```python
from build123d import *

# Parameters (mm, degrees)
SKETCH_1_W          = 20
SKETCH_1_H          = 20
EXTRUDE_1_DEPTH     = 5
SKETCH_2_R          = 1.525
CUT_EXTRUDE_1_DEPTH = 10
CUT_EXTRUDE_2_DEPTH = 6
FILLET_2_R          = 2


with BuildPart() as part:
    # 草图1 → 凸台-拉伸1 (new body)
    with BuildSketch(Plane(origin=(0, 0, 0), x_dir=(1, 0, 0), z_dir=(0, 1, 0))):
        Rectangle(SKETCH_1_W, SKETCH_1_H)
    extrude(amount=EXTRUDE_1_DEPTH)

    # 草图2 → 切除-拉伸1 (cut)
    with BuildSketch(Plane(origin=(0, 5, 0), x_dir=(1, 0, 0), z_dir=(0, 1, 0))):
        with Locations((-7.5, -7)):
            Circle(SKETCH_2_R)
        with Locations((7.5, -7)):
            Circle(SKETCH_2_R)
    extrude(amount=-CUT_EXTRUDE_1_DEPTH, mode=Mode.SUBTRACT)

    # 草图3 → 切除-拉伸2 (cut, through all)
    with BuildSketch(Plane(origin=(0, 5, 0), x_dir=(1, 0, 0), z_dir=(0, 1, 0))):
        Polygon((-10, 10), (-10, 0.585811222), (10, 7.865215908), (10, 10), align=None)
    extrude(amount=-CUT_EXTRUDE_2_DEPTH, mode=Mode.SUBTRACT)

    # 圆角2
    fillet_2_edges = [part.edges().sort_by_distance(p)[0] for p in [
        (-10, 2.5, -0.585811222),
        (10, 2.5, -7.865215908),
        (10, 2.5, 10),
        (-10, 2.5, 10),
    ]]
    fillet(fillet_2_edges, radius=FILLET_2_R)


solid = part.part
```
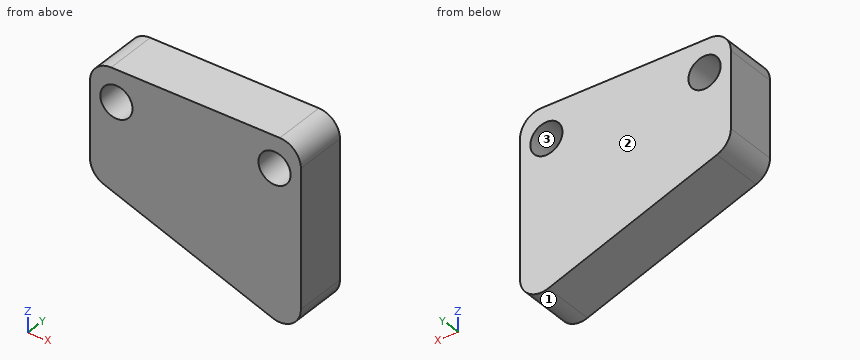
Check sheet for the modelled part. Datum: model origin and axes. Units: mm. Face numbers are marked on the shaded views. Coordinates: 2 decimals unless noted, no trailing zeros. Order: outer loops, then holes, each group sorted by start corner. A loop starts at its lowest first (then second) coordinate and runs counter-clockwise, first axis right, second up. Notation, with made-up numbers: (74.25, 62.5) -> (82.25, 62.5) arc R13 cw to (82.25, 76.5) -> close; hole circle Ø6 at (45.25, 45). An arc over 180 degrees is marked (long way). Write item = value, one per line. Start each with the question number.
1) Cross-section at C-C (x = -7.5). Enter the section's corners in (y, z) (3 decimals), then the cut area to 3 significant figures.
2) Cross-section at D-D (x = -2.75). Enter the section's corners in (y, z), then the cut area to 3 significant figures.
3) Mould release check, pull along Z, two halves, no side actions. Record for the marked faces 1, 2 and 3: +Z half, -Z half, draft (parallel to the pull), parting line (faces both ways), or undercut.
4) Material ranges on L1, parallel to X at y = 2.6, z = 7 (3 decimals); L2, parallel to X at y = 0.4, z = 6; L3, parallel to Z at x = 7.5, y = 3.5 (3 decimals), recorded low to high.
5) Cross-section at A-A (z = 7). Enter the section's corners in (x, y) (3 decimals), then the cut area to 3 significant figures.
6) Cross-section at B-B (y = 4.05). Enter the section's corners in (x, z) (3 decimals).
Ans:
q1.outline = (0, -1.496) -> (5, -1.496) -> (5, 5.475) -> (0, 5.475) -> close; (0, 8.525) -> (5, 8.525) -> (5, 10) -> (0, 10) -> close
q1.area = 42.2 mm²
q2.outline = (0, -3.22) -> (5, -3.22) -> (5, 10) -> (0, 10) -> close
q2.area = 66.1 mm²
q3.face_1 = -Z half
q3.face_2 = draft
q3.face_3 = undercut
q4.L1 = -10 to -9.025, -5.975 to 5.975, 9.025 to 10
q4.L2 = -10 to -8.65, -6.35 to 6.35, 8.65 to 10
q4.L3 = -6.945 to 5.475, 8.525 to 10
q5.outline = (-10, 0) -> (-9.025, 0) -> (-9.025, 5) -> (-10, 5) -> close; (-5.975, 0) -> (5.975, 0) -> (5.975, 5) -> (-5.975, 5) -> close; (9.025, 0) -> (10, 0) -> (10, 5) -> (9.025, 5) -> close
q5.area = 69.5 mm²
q6.outline = (-10, 0.815) arc R2 ccw to (-8.684, -1.065) -> (7.316, -6.888) arc R2 ccw to (10, -5.009) -> (10, 8) arc R2 ccw to (8, 10) -> (-8, 10) arc R2 ccw to (-10, 8) -> close; hole circle Ø3.05 at (-7.5, 7); hole circle Ø3.05 at (7.5, 7)
